Read the model definition and answer for the solid it produces. Units are mm, in the model's axes. Give positions to 0.01 mm unless a question says otherwise; leave off trailing zeros. Order: outer loops, then holes, each group sorted by start corner. A loop starts at its lowest first (then second) coordinate and runs counter-clockwise, first axis right, second up. Notation, with made-up numbers: (-6.5, 55.5) -> (25.5, 55.5) arc R9 cw to (25.5, 69.5) -> close; hole circle Ø6 at (4, 79). An arc over 180 degrees is marked (long way). Use one line per item in the form item = value.
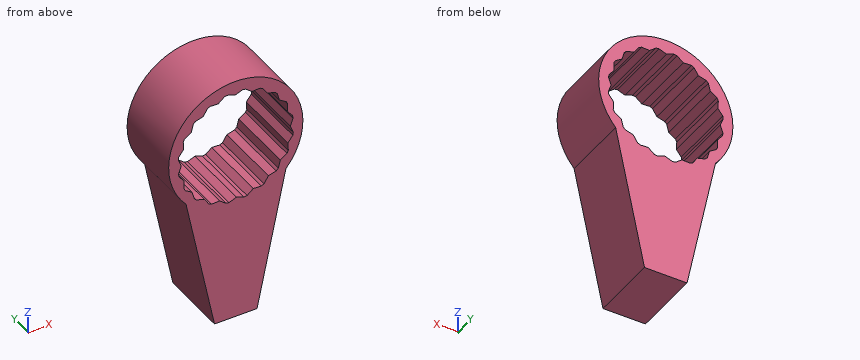
```python
from build123d import *

# Parameters (mm, degrees)
Y_KSEKLIK_EKSTR_ZYON1_DEPTH = 3
KES_EKSTR_ZYON1_DEPTH       = 3


with BuildPart() as part:
    # Çizim2 → Yükseklik-Ekstrüzyon1 (new body)
    with BuildSketch(Plane(origin=(0, 0, 0), x_dir=(1, 0, 0), z_dir=(0, 1, 0))):
        with BuildLine():
            Line((-2.149165658, 1.947071384), (-0.918653313, 7.910801403))
            Line((-0.918653313, 7.910801403), (0.918505018, 7.890194196))
            Line((0.918505018, 7.890194196), (2.165891081, 1.928449073))
            ThreePointArc((2.165891081, 1.928449073), (-0.012515293, -2.899972994), (-2.149165658, 1.947071384))
        make_face()
    extrude(amount=Y_KSEKLIK_EKSTR_ZYON1_DEPTH)

    # Çizim3 → Kes-Ekstrüzyon1 (cut)
    with BuildSketch(Plane(origin=(0, 3, -0.083225357), x_dir=(1, 0, 0), z_dir=(0, 1, 0))):
        Polygon((-1.696920921, 1.837383666), (-1.792135812, 1.744599792), (-1.88879277, 1.410713864), (-2.181417312, 1.223115215), (-2.243300262, 1.105449488), (-2.232050065, 0.758036458), (-2.452381372, 0.489193583), (-2.474874845, 0.358163944), (-2.356818742, 0.031231019), (-2.48328925, -0.292539866), (-2.464191429, -0.424107324), (-2.250885573, -0.69855767), (-2.271115468, -1.045563617), (-2.212295781, -1.164790154), (-1.924620035, -1.359892809), (-1.836629074, -1.696166458), (-1.743845201, -1.791381349), (-1.409959273, -1.888038307), (-1.222360623, -2.180662849), (-1.104694896, -2.242545799), (-0.757281866, -2.231295602), (-0.488438992, -2.451626909), (-0.357409352, -2.474120382), (-0.030476428, -2.356064279), (0.293294458, -2.482534787), (0.424861916, -2.463436966), (0.699312262, -2.25013111), (1.046318209, -2.270361005), (1.165544745, -2.211541317), (1.360647401, -1.923865572), (1.696921049, -1.835874611), (1.792135941, -1.743090737), (1.888792899, -1.409204809), (2.181417441, -1.22160616), (2.24330039, -1.103940433), (2.232050194, -0.756527403), (2.4523815, -0.487684528), (2.474874973, -0.356654889), (2.35681887, -0.029721965), (2.483289379, 0.294048921), (2.464191557, 0.425616379), (2.250885702, 0.700066725), (2.271115596, 1.047072672), (2.212295909, 1.166299208), (1.924620164, 1.361401864), (1.836629202, 1.697675512), (1.743845329, 1.792890404), (1.409959401, 1.889547362), (1.222360751, 2.182171904), (1.104695025, 2.244054853), (0.757281994, 2.232804657), (0.48843912, 2.453135964), (0.357409481, 2.475629437), (0.030476556, 2.357573334), (-0.29329433, 2.484043842), (-0.424861787, 2.464946021), (-0.699312133, 2.251640165), (-1.04631808, 2.27187006), (-1.165544617, 2.213050372), (-1.360647273, 1.925374627), align=None)
    extrude(amount=-KES_EKSTR_ZYON1_DEPTH, mode=Mode.SUBTRACT)


solid = part.part
```
Item 1: The part is cut by section A-A on z = -5. Give the vertices of the cut face in (x, y).
Checks:
outline = (-1.52, 0) -> (1.52, 0) -> (1.52, 3) -> (-1.52, 3) -> close
Item 2: Given pin 1 Ø1 at (y, z) = (1, -5.5) entering from +X, flat-ended and moving along its own axis, determine where the tip first touches the part or whether it passes through.
Checks:
pin_1 = 1.52
Item 3: Straight lines are drawn through the part: L1, parallel to Z at x = -0.85, y = 1; L2, parallel to Z at x = -0.5, y = 0.2; L3, parallel to X at y = 0.25, z = 2.5. For each, find the intervals that lie inside material, in ascending order. Write a range as from..to.
Checks:
L1 = -7.91..-2.34, 2.15..2.77
L2 = -7.91..-2.49, 2.36..2.86
L3 = -1.47..1.47
